```python
from build123d import *

# Parameters (mm, degrees)
SKETCH9_R           = 2.305
SKETCH9_R_2         = 1.778
BOSS_EXTRUDE1_DEPTH = 6.35


with BuildPart() as part:
    # Sketch9 → Boss-Extrude1 (new body)
    with BuildSketch(Plane.XY):
        with BuildLine():
            Line((19.05, 0), (69.85, 0))
            ThreePointArc((69.85, 0), (79.428440233, 11.849261314), (69.85, 23.698522628))
            Line((69.85, 23.698522628), (19.05, 23.698522628))
            Line((19.05, 23.698522628), (13.97, 23.698522628))
            ThreePointArc((13.97, 23.698522628), (4.391559767, 11.849261314), (13.97, 0))
            Line((13.97, 0), (19.05, 0))
        make_face()
        with Locations((44.45, 11.849261314)):
            Circle(SKETCH9_R, mode=Mode.SUBTRACT)
        with Locations((67.31, 11.849261314)):
            Circle(SKETCH9_R_2, mode=Mode.SUBTRACT)
        with Locations((21.59, 11.849261314)):
            Circle(SKETCH9_R_2, mode=Mode.SUBTRACT)
    extrude(amount=BOSS_EXTRUDE1_DEPTH)


solid = part.part
```
Model file for the job. Use its own axes, mm. Give positions to 0.01 mm unless a question says otherwise; leave off trailing zeros. Write each loop counter-clockwise with the first axis right and the second up, starting at its lowest first coordinate (ties: lowest second). Pieces come first, ordered by that corner, then holes. Notation, with made-up numbers: (20, 64) - (36, 64) arc R17 ccw to (36, 83) - close; hole circle Ø11 at (13, -11). An arc over 180 degrees is marked (long way). One line per question, with ' | ' between items. Start each with the question number.
(1) Slice it at B-B on z = 1.25. Write the cut outline in (x, y) (3 decimals), plus the area to 3 significant figures.
(2) Slice it at D-D on y = 3. Write the cut outline in (x, z), plus the area to 3 significant figures.
(3) Slice it at A-A on x = 44.45. Write the cut outline in (y, z), plus the area to 3 significant figures.
(4) Wall check: line 1 along X through (y, z) = (12.25, 3.25); line 2 along Y through (x, z) = (67.31, 5.25); line 3 along Y through (x, z) = (44.45, 2.5). Give the ranges that are in metal, low to high. Write a range as from..to.
(5) Pin check, flat tips, straight feed: P1, Ø3, axis at y = 7.5, z = 4.5, coming from the -X side; P2, Ø8, axis at x = 61.5, y = 16, coming from the -Z side; P3, Ø2, axis at y = 19.5, z = 3.5, coming from the +X side; P4, Ø3, axis at x = 44.45, y = 11.85, coming from the -Z side. Stop position of each tip, or through.
(6) Two-plate mould, pull along Y, no slides. Class faces 1 (the face through (41, 12, 6.35)), 2 (the face through (42, 23.699, 3)), 3 (the face through (45.69, 13.79, 3.13)), 4 (the face through (79.426, 11.619, 3.131)): +Y half, -Y half, draft (parallel to the pull), parting line (faces both ways), or undercut.
(7) Slice it at C-C on x = 21.59. Write the cut outline in (y, z).
Results below:
1) outline: (13.97, 0) - (69.85, 0) arc R12.118 ccw to (69.85, 23.699) - (13.97, 23.699) arc R12.118 ccw to start; hole circle Ø3.556 at (21.59, 11.849); hole circle Ø4.61 at (44.45, 11.849); hole circle Ø3.556 at (67.31, 11.849) | area: 1,630 mm^2
2) outline: (8.23, 0) - (75.59, 0) - (75.59, 6.35) - (8.23, 6.35) - close | area: 428 mm^2
3) outline: (0, 0) - (9.54, 0) - (9.54, 6.35) - (0, 6.35) - close; (14.15, 0) - (23.7, 0) - (23.7, 6.35) - (14.15, 6.35) - close | area: 121 mm^2
4) line 1: 4.4..19.86, 23.32..42.18, 46.72..65.58, 69.04..79.42 | line 2: 0..10.07, 13.63..23.7 | line 3: 0..9.54, 14.15..23.7
5) P1: x = 4.73 | P2: z = 0 | P3: x = 77.44 | P4: through
6) face 1: draft | face 2: +Y half | face 3: undercut | face 4: parting line
7) outline: (0, 0) - (10.07, 0) - (10.07, 6.35) - (0, 6.35) - close; (13.63, 0) - (23.7, 0) - (23.7, 6.35) - (13.63, 6.35) - close
